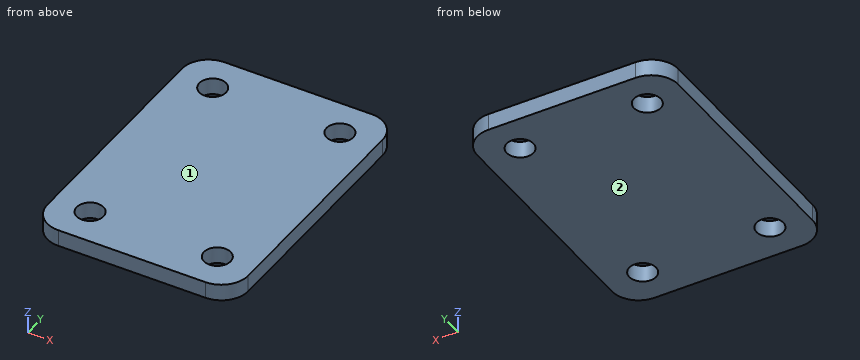
```python
from build123d import *

# Parameters (mm, degrees)
SKETCH2_W               = 138
SKETCH2_H               = 42
SKETCH2_R               = 2
SKETCH2_R_2             = 3.5
SKETCH2_R_3             = 8.5
BOSS_EXTRUDE1_DEPTH     = 2.38125
SKETCH3_R               = 4
SKETCH3_R_2             = 2
CUT_EXTRUDE1_DEPTH      = 4
SKETCH4_R               = 3.175
SKETCH4_R_2             = 2
BOSS_EXTRUDE2_DEPTH     = 17.9
SKETCH6_R               = 2
CUT_EXTRUDE2_DEPTH      = 10
BOSS_EXTRUDE3_DEPTH     = 4.7625
SKETCH7_R               = 3.175
BOSS_EXTRUDE4_DEPTH     = 17.9
FILLET1_R               = 6.35
BOSS_EXTRUDE5_START     = -27.425
BOSS_EXTRUDE5_DEPTH     = 27.425
CUT_EXTRUDE4_START      = -4
SKETCH9_R               = 4
CUT_EXTRUDE4_DEPTH      = 4
SKETCH10_R              = 11.00455
CUT_EXTRUDE5_DEPTH      = 2.5
CUT_EXTRUDE6_DEPTH      = 123.578796086
CUT_EXTRUDE6_DEPTH_BACK = 123.578796086
SKETCH11_R              = 1.65
SKETCH12_R              = 2
BOSS_EXTRUDE6_DEPTH     = 2.5


with BuildPart() as part:
    # Sketch2 → Boss-Extrude1 (new, symmetric)
    with BuildSketch(Plane.XY):
        with Locations((48, 0)):
            Rectangle(SKETCH2_W, SKETCH2_H)
        with Locations(Location((34, -15.5, 0), (0, 0, 180))):
            Circle(SKETCH2_R, mode=Mode.SUBTRACT)
        with Locations(Location((34, 15.5, 0), (0, 0, 180))):
            Circle(SKETCH2_R, mode=Mode.SUBTRACT)
        with Locations(Location((0, 0, 0), (0, 0, 180))):
            Circle(SKETCH2_R_2, mode=Mode.SUBTRACT)
        with Locations(Location((60, 0, 0), (0, 0, 180))):
            Circle(SKETCH2_R_3, mode=Mode.SUBTRACT)
    boss_extrude1 = extrude(amount=BOSS_EXTRUDE1_DEPTH, both=True)

    # Sketch3 → Cut-Extrude1 (cut)
    # profile 1 of 6: a face of its own
    with BuildSketch(Plane(origin=(0, 0, -2.38125), x_dir=(-1, 0, 0), z_dir=(0, 0, -1))):
        with Locations((-34, -15.5)):
            Circle(SKETCH3_R)
    # profile 2 of 6: a face of its own
    with BuildSketch(Plane(origin=(0, 0, -2.38125), x_dir=(-1, 0, 0), z_dir=(0, 0, -1))):
        with Locations((-34, 15.5)):
            Circle(SKETCH3_R)
        with Locations((-34, 15.5)):
            Circle(SKETCH3_R_2, mode=Mode.SUBTRACT)
    # profile 3 of 6: a face of its own
    with BuildSketch(Plane(origin=(0, 0, -2.38125), x_dir=(-1, 0, 0), z_dir=(0, 0, -1))):
        with Locations((-15.5, 15.5)):
            Circle(SKETCH3_R)
    # profile 4 of 6: a face of its own
    with BuildSketch(Plane(origin=(0, 0, -2.38125), x_dir=(-1, 0, 0), z_dir=(0, 0, -1))):
        with Locations((15.5, 15.5)):
            Circle(SKETCH3_R)
    # profile 5 of 6: a face of its own
    with BuildSketch(Plane(origin=(0, 0, -2.38125), x_dir=(-1, 0, 0), z_dir=(0, 0, -1))):
        with Locations((-15.5, -15.5)):
            Circle(SKETCH3_R)
    # profile 6 of 6: a face of its own
    with BuildSketch(Plane(origin=(0, 0, -2.38125), x_dir=(-1, 0, 0), z_dir=(0, 0, -1))):
        with Locations((15.5, -15.5)):
            Circle(SKETCH3_R)
    extrude(amount=-CUT_EXTRUDE1_DEPTH, mode=Mode.SUBTRACT)

    # Sketch4 → Boss-Extrude2 (add)
    # profile 1 of 2: a face of its own
    with BuildSketch(Plane(origin=(0, 0, -2.38125), x_dir=(-1, 0, 0), z_dir=(0, 0, -1))):
        with Locations(Location((-111.5, -15.5, 0), (0, 0, 180))):
            Circle(SKETCH4_R)
        with Locations(Location((-111.5, -15.5, 0), (0, 0, 180))):
            Circle(SKETCH4_R_2, mode=Mode.SUBTRACT)
    # profile 2 of 2: a face of its own
    with BuildSketch(Plane(origin=(0, 0, -2.38125), x_dir=(-1, 0, 0), z_dir=(0, 0, -1))):
        with Locations(Location((-111.5, 15.5, 0), (0, 0, 180))):
            Circle(SKETCH4_R)
        with Locations(Location((-111.5, 15.5, 0), (0, 0, 180))):
            Circle(SKETCH4_R_2, mode=Mode.SUBTRACT)
    extrude(amount=BOSS_EXTRUDE2_DEPTH)

    # Sketch6 → Cut-Extrude2 (cut)
    with BuildSketch(Plane(origin=(0, 0, -2.38125), x_dir=(-1, 0, 0), z_dir=(0, 0, -1))):
        with Locations((-15.5, 15.5)):
            Circle(SKETCH6_R)
        with Locations((15.5, 15.5)):
            Circle(SKETCH6_R)
        with Locations((15.5, -15.5)):
            Circle(SKETCH6_R)
        with Locations((-15.5, -15.5)):
            Circle(SKETCH6_R)
    extrude(amount=-CUT_EXTRUDE2_DEPTH, mode=Mode.SUBTRACT)

    # Sketch5 → Boss-Extrude3 (add)
    with BuildSketch(Plane(origin=(0, 0, -2.38125), x_dir=(-1, 0, 0), z_dir=(0, 0, -1))):
        with BuildLine():
            Line((21, -21), (27.208091957, -0.938604379))
            ThreePointArc((27.208091957, -0.938604379), (27.35, 0), (27.208091957, 0.938604379))
            Line((27.208091957, 0.938604379), (21, 21))
            Line((21, 21), (21, -21))
        make_face()
    boss_extrude3 = extrude(amount=-BOSS_EXTRUDE3_DEPTH)

    # Mirror2: Boss-Extrude1, Boss-Extrude3 across plane
    add(boss_extrude1.mirror(Plane(origin=(0, 0, -11.33125), x_dir=(1, 0, 0), z_dir=(0, 0, -1))))
    add(boss_extrude3.mirror(Plane(origin=(0, 0, -11.33125), x_dir=(1, 0, 0), z_dir=(0, 0, -1))))

    # Sketch7 → Boss-Extrude4 (add)
    with BuildSketch(Plane.XY.offset(-20.28125)):
        with Locations(Location((-24.175, 0, 0), (0, 0, 197.194924512))):
            Circle(SKETCH7_R)
    extrude(amount=BOSS_EXTRUDE4_DEPTH)

    # Fillet1
    fillet1_edges = [part.edges().sort_by_distance(p)[0] for p in [
        (117, 21, -22.6625),
        (117, -21, -22.6625),
        (-21, -21, -22.6625),
        (-21, 21, -22.6625),
        (117, -21, 0),
        (-21, -21, 0),
        (-21, 21, 0),
        (117, 21, 0),
    ]]
    fillet(fillet1_edges, radius=FILLET1_R)

    # Sketch8 → Boss-Extrude5 (add)
    with BuildSketch(Plane(origin=(0, 0, -25.04375), x_dir=(-1, 0, 0), z_dir=(0, 0, -1)).offset(BOSS_EXTRUDE5_START)):
        with BuildLine():
            ThreePointArc((3.175, 21), (0, 24.175), (-3.175, 21))
            Line((-3.175, 21), (3.175, 21))
        make_face()
        with BuildLine():
            Line((3.175, -21), (-3.175, -21))
            ThreePointArc((-3.175, -21), (0, -24.175), (3.175, -21))
        make_face()
    extrude(amount=BOSS_EXTRUDE5_DEPTH)

    # Sketch9 → Cut-Extrude4 (cut)
    with BuildSketch(Plane.XY.offset(-20.28125).offset(CUT_EXTRUDE4_START)):
        with Locations(Location((34, -15.5, 0), (0, 0, 180))):
            Circle(SKETCH9_R)
        with Locations(Location((34, 15.5, 0), (0, 0, 180))):
            Circle(SKETCH9_R)
    extrude(amount=CUT_EXTRUDE4_DEPTH, mode=Mode.SUBTRACT)

    # Sketch10 → Cut-Extrude5 (cut)
    with BuildSketch(Plane.XY.offset(2.38125)):
        Circle(SKETCH10_R)
    extrude(amount=-CUT_EXTRUDE5_DEPTH, mode=Mode.SUBTRACT)

    # Sketch11 → Cut-Extrude6 (cut, two sides: drawn at the far end of the back side and taken through both)
    with BuildSketch(Plane.XY.offset(2.38125).offset(-CUT_EXTRUDE6_DEPTH_BACK)):
        with Locations((50.5, 15.5)):
            Circle(SKETCH11_R)
        with Locations(Location((69.5, 15.5, 0), (0, 0, 180))):
            Circle(SKETCH11_R)
        with Locations((69.5, -15.5)):
            Circle(SKETCH11_R)
        with Locations(Location((50.5, -15.5, 0), (0, 0, 180))):
            Circle(SKETCH11_R)
    extrude(amount=CUT_EXTRUDE6_DEPTH + CUT_EXTRUDE6_DEPTH_BACK, mode=Mode.SUBTRACT)


with BuildPart() as body_2:
    # Sketch12 → Boss-Extrude6 (new body)
    with BuildSketch(Plane.XY.offset(2.38125)):
        with BuildLine():
            Line((49, 21), (71, 21))
            ThreePointArc((71, 21), (73.828427125, 19.828427125), (75, 17))
            Line((75, 17), (75, -17))
            ThreePointArc((75, -17), (73.828427125, -19.828427125), (71, -21))
            Line((71, -21), (49, -21))
            ThreePointArc((49, -21), (46.171572875, -19.828427125), (45, -17))
            Line((45, -17), (45, 17))
            ThreePointArc((45, 17), (46.171572875, 19.828427125), (49, 21))
        make_face()
        with Locations((50.5, 15.5)):
            Circle(SKETCH12_R, mode=Mode.SUBTRACT)
        with Locations(Location((69.5, 15.5, 0), (0, 0, 180))):
            Circle(SKETCH12_R, mode=Mode.SUBTRACT)
        with Locations((69.5, -15.5)):
            Circle(SKETCH12_R, mode=Mode.SUBTRACT)
        with Locations(Location((50.5, -15.5, 0), (0, 0, 180))):
            Circle(SKETCH12_R, mode=Mode.SUBTRACT)
    extrude(amount=BOSS_EXTRUDE6_DEPTH)


solid = body_2.part
```
Geometry check sheet. Reference: the model listing, model coordinates, mm. Face numbers are marked on the shaded views. Give positions to 0.01 mm unless a question says otherwise; leave off trailing zeros. Loops run counter-clockwise (first coordinate to the right, second up) from the corner with the lowest first, then second, coordinate; pieces in that order, holes last. Notation, with made-up numbers: M 3,-33 L 22,-33 A22 ccw 22,-4 Z; hole C 17.25,84 d6. An arc over 180 degrees is marked long. Answer as CSV lines item,"result".
Item 1: Material ranges on line 1 (Y direction, x = 50.5, z = 3.55); line 2 (Y direction, x = 68.5, z = 3); line 3 (X direction, y = 17, z = 3.6), recorded low to high.
Values:
line 1,"y = -21 to -17.5, -13.5 to 13.5, 17.5 to 21"
line 2,"y = -21 to -17.23, -13.77 to 13.77, 17.23 to 21"
line 3,"x = 45 to 49.18, 51.82 to 68.18, 70.82 to 75"
Item 2: Release check for a two-part mould opening along Z. For the marked faces 1 and 2 record: pulls with the +Z half, pulls with the -Z half, needs draft (parallel to the pull), parting line crosses it, or undercut.
Values:
face 1,"pulls with the +Z half"
face 2,"pulls with the -Z half"
Item 3: Cross-section at A-A on z = 3.2. Record the cut outline in (x, y), and give its area (3 significant figures).
Values:
outline,"M 45,-17 A4 ccw 49,-21 L 71,-21 A4 ccw 75,-17 L 75,17 A4 ccw 71,21 L 49,21 A4 ccw 45,17 Z; hole C 50.5,-15.5 d4; hole C 50.5,15.5 d4; hole C 69.5,-15.5 d4; hole C 69.5,15.5 d4"
area,"1,200 mm²"
Item 4: Depth check by flat-ended pin: P1, Ø4.5, axis at x = 69.5, y = 15.5, coming from the +Z side. Enter the tip coordinate at first touch or a pass-through.
Values:
P1,"stops at z = 4.88"
Item 5: Cross-section at B-B on x = 69.5. Record the cut outline in (y, z), and give its area (3 significant figures).
Values:
outline,"M -21,2.38 L -17.5,2.38 L -17.5,4.88 L -21,4.88 Z; M -13.5,2.38 L 13.5,2.38 L 13.5,4.88 L -13.5,4.88 Z; M 17.5,2.38 L 21,2.38 L 21,4.88 L 17.5,4.88 Z"
area,"85.0 mm²"
